```python
from build123d import *

# Parameters (mm, degrees)
SKETCH1_R           = 3
SKETCH1_R_2         = 1.7
SKETCH1_R_3         = 26
BOSS_EXTRUDE1_DEPTH = 6.35


with BuildPart() as part:
    # Sketch1 → Boss-Extrude1 (new body)
    with BuildSketch(Plane(origin=(0, 0, 0), x_dir=(1, 0, 0), z_dir=(0, 1, 0))):
        with BuildLine():
            Line((0, 46.5), (500, 46.5))
            ThreePointArc((500, 46.5), (546.5, 0), (500, -46.5))
            Line((500, -46.5), (0, -46.5))
            ThreePointArc((0, -46.5), (-46.5, 0), (0, 46.5))
        make_face()
        with Locations(Location((-16, 0, 0), (0, 0, 270))):
            Circle(SKETCH1_R, mode=Mode.SUBTRACT)
        with Locations(Location((-11.313708499, 11.313708499, 0), (0, 0, 270))):
            Circle(SKETCH1_R, mode=Mode.SUBTRACT)
        with Locations(Location((0, 16, 0), (0, 0, 270))):
            Circle(SKETCH1_R, mode=Mode.SUBTRACT)
        with Locations(Location((11.313708499, 11.313708499, 0), (0, 0, 270))):
            Circle(SKETCH1_R, mode=Mode.SUBTRACT)
        with Locations(Location((16, 0, 0), (0, 0, 270))):
            Circle(SKETCH1_R, mode=Mode.SUBTRACT)
        with Locations(Location((11.313708499, -11.313708499, 0), (0, 0, 270))):
            Circle(SKETCH1_R, mode=Mode.SUBTRACT)
        with Locations(Location((537.25, 0, 0), (0, 0, 270))):
            Circle(SKETCH1_R_2, mode=Mode.SUBTRACT)
        with Locations(Location((530.13588304, -21.895000648, 0), (0, 0, 270))):
            Circle(SKETCH1_R_2, mode=Mode.SUBTRACT)
        with Locations(Location((511.51088304, -35.426855232, 0), (0, 0, 270))):
            Circle(SKETCH1_R_2, mode=Mode.SUBTRACT)
        with Locations(Location((488.48911696, -35.426855232, 0), (0, 0, 270))):
            Circle(SKETCH1_R_2, mode=Mode.SUBTRACT)
        with Locations(Location((469.86411696, -21.895000648, 0), (0, 0, 270))):
            Circle(SKETCH1_R_2, mode=Mode.SUBTRACT)
        with Locations(Location((462.75, 0, 0), (0, 0, 270))):
            Circle(SKETCH1_R_2, mode=Mode.SUBTRACT)
        with Locations(Location((469.86411696, 21.895000648, 0), (0, 0, 270))):
            Circle(SKETCH1_R_2, mode=Mode.SUBTRACT)
        with Locations(Location((488.48911696, 35.426855232, 0), (0, 0, 270))):
            Circle(SKETCH1_R_2, mode=Mode.SUBTRACT)
        with Locations(Location((511.51088304, 35.426855232, 0), (0, 0, 270))):
            Circle(SKETCH1_R_2, mode=Mode.SUBTRACT)
        with Locations(Location((530.13588304, 21.895000648, 0), (0, 0, 270))):
            Circle(SKETCH1_R_2, mode=Mode.SUBTRACT)
        with Locations(Location((500, 0, 0), (0, 0, 270))):
            Circle(SKETCH1_R_3, mode=Mode.SUBTRACT)
        with Locations(Location((0, -16, 0), (0, 0, 270))):
            Circle(SKETCH1_R, mode=Mode.SUBTRACT)
        with Locations(Location((-11.313708499, -11.313708499, 0), (0, 0, 270))):
            Circle(SKETCH1_R, mode=Mode.SUBTRACT)
    extrude(amount=BOSS_EXTRUDE1_DEPTH)


solid = part.part
```
The model under review builds one solid part; all positions refer to its coordinate system, in mm. Round coordinates to 2 decimals unless told otherwise and drop trailing zeros. Use a Markdown table: item, result.
Q1. Mouldability with a two-part tool opening along Z and no side actions: class faces 1 (the flat face through (254, 0, -1)), 2 (the cylindrical face through (517.572, 3.131, -19.163)), 3 (the cylindrical face through (-46.49, 3.13, 1.02)) as +Z half, -Z half, draft (parallel to the pull), parting line (faces both ways), or undercut.
Values:
| item | result |
|---|---|
| face 1 | draft |
| face 2 | undercut |
| face 3 | parting line |
Q2. We need section A-A on y = 5.25. State how many separate pieces and enclosed holes the cut face has, then the cut area to 3 significant figures.
Values:
| item | result |
|---|---|
| separate pieces | 1 |
| enclosed holes | 19 |
| area | 50,900 mm^2 |
Q3. For line 1 (X direction, y = 4, z = 0); line 2 (X direction, y = 4.5, z = 9.5); line 3 (X direction, y = 4.5, z = -9), list the stretches that pass through material, from the lowest coordinate up.
Values:
| item | result |
|---|---|
| line 1 | x = -46.5 to -19, -13 to 13, 19 to 461.05, 464.45 to 474, 526 to 535.55, 538.95 to 546.5 |
| line 2 | x = -45.52 to -13.7, -8.92 to 8.92, 13.7 to 475.8, 524.2 to 545.52 |
| line 3 | x = -45.62 to -13.22, -9.4 to 9.4, 13.22 to 475.61, 524.39 to 545.62 |
Q4. Clearance check with a flat-ended pin moving along its axis: P1, Ø2, axis at y = 5, z = 0.5, coming from the +X side. State where the tip first meets the part, or that it passes through.
Values:
| item | result |
|---|---|
| P1 | stops at x = 546.5 |
